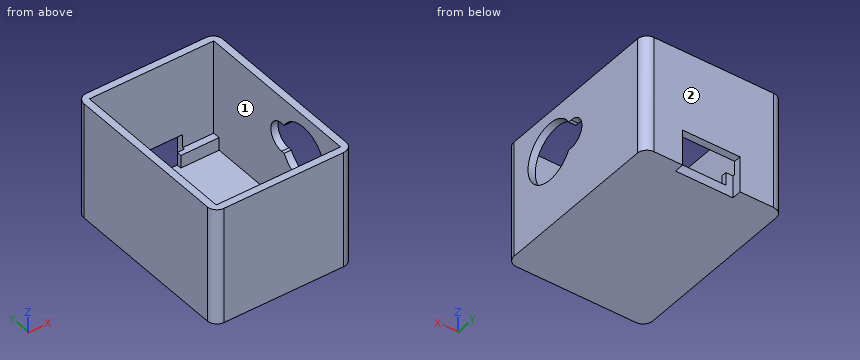
```python
from build123d import *

# Parameters (mm, degrees)
SKETCH_1_W               = 29
SKETCH_1_H               = 38.5
EXTRUDE_1_DEPTH          = 24
SHELL_1_T                = -1.5
SKETCH_7_W               = 26
SKETCH_7_H               = 5.5
EXTRUDE_7_DEPTH          = 2.5
SKETCH_5_W               = 2.7
SKETCH_5_H               = 1.5
EXTRUDE_8_DEPTH          = 8
SKETCH_6_W               = 2.7
SKETCH_6_H               = 1.5
EXTRUDE_9_DEPTH          = 9
SKETCH_9_W               = 29
SKETCH_9_H               = 38.5
EXTRUDE_10_DEPTH         = 0.5
FILLET_3_R               = 2
CUT_EXTRUDE_8_DEPTH      = 1.5
CUT_EXTRUDE_8_DEPTH_BACK = 7
SKETCH_2_W               = 12
SKETCH_2_H               = 2
SKETCH_10_R              = 3
SKETCH_10_R_2            = 6.072147162
CUT_EXTRUDE_9_DEPTH      = 1.5


with BuildPart() as part:
    # 草图1 → 凸台-拉伸1 (new body)
    with BuildSketch(Plane.XY):
        with Locations((14.5, -19.25)):
            Rectangle(SKETCH_1_W, SKETCH_1_H)
    extrude(amount=EXTRUDE_1_DEPTH)

    # 抽壳1
    shell_1_openings = [part.faces().sort_by_distance(p)[0] for p in [
        (14.5, -19.25, 24),
    ]]
    offset(amount=SHELL_1_T, openings=shell_1_openings, kind=Kind.INTERSECTION)

    # 草图7 → 凸台-拉伸7 (add)
    with BuildSketch(Plane.XY.offset(1.5)):
        with Locations((14.5, -34.25)):
            Rectangle(SKETCH_7_W, SKETCH_7_H)
    extrude(amount=EXTRUDE_7_DEPTH)

    # 草图5 → 凸台-拉伸8 (add)
    with BuildSketch(Plane.ZY.offset(-27.5)):
        with Locations((2.85, -2.25)):
            Rectangle(SKETCH_5_W, SKETCH_5_H)
    extrude(amount=EXTRUDE_8_DEPTH)

    # 草图6 → 凸台-拉伸9 (add)
    with BuildSketch(Plane(origin=(1.5, 0, 0), x_dir=(0, 0, -1), z_dir=(1, 0, 0))):
        with Locations((-2.85, -2.25)):
            Rectangle(SKETCH_6_W, SKETCH_6_H)
    extrude(amount=EXTRUDE_9_DEPTH)

    # 草图9 → 凸台-拉伸10 (add)
    with BuildSketch(Plane(origin=(0, 0, 0), x_dir=(-1, 0, 0), z_dir=(0, 0, -1))):
        with Locations((-14.5, -19.25)):
            Rectangle(SKETCH_9_W, SKETCH_9_H)
    extrude(amount=EXTRUDE_10_DEPTH)

    # 圆角3
    fillet_3_edges = [part.edges().sort_by_distance(p)[0] for p in [
        (0, 0, 11.75),
        (29, 0, 11.75),
        (29, -38.5, 11.75),
        (0, -38.5, 11.75),
    ]]
    fillet(fillet_3_edges, radius=FILLET_3_R)

    # 草图2 → 切除-拉伸8 (cut, two sides: drawn at the far end of the back side and taken through both)
    with BuildSketch(Plane(origin=(0, 0, 0), x_dir=(-1, 0, 0), z_dir=(0, 0, -1)).offset(-CUT_EXTRUDE_8_DEPTH_BACK)):
        with Locations((-15, -1)):
            Rectangle(SKETCH_2_W, SKETCH_2_H)
    extrude(amount=CUT_EXTRUDE_8_DEPTH + CUT_EXTRUDE_8_DEPTH_BACK, mode=Mode.SUBTRACT)

    # 草图10 → 切除-拉伸9 (cut)
    with BuildSketch(Plane(origin=(29, 0, 0), x_dir=(0, 0, -1), z_dir=(1, 0, 0))):
        with Locations((-15.5, -20.5)):
            Circle(SKETCH_10_R)
        with Locations((-15.5, -26.5)):
            Circle(SKETCH_10_R_2)
        with BuildLine():
            ThreePointArc((-18.422516621, -21.177419071), (-18.48056621, -20.840917978), (-18.5, -20.5))
            Line((-18.5, -20.5), (-18.5, -21.220703536))
            ThreePointArc((-18.5, -21.220703536), (-18.461337395, -21.198919734), (-18.422516621, -21.177419071))
        make_face()
        with BuildLine():
            Line((-12.5, -21.220703536), (-12.5, -20.5))
            ThreePointArc((-12.5, -20.5), (-12.51943379, -20.840917978), (-12.577483379, -21.177419071))
            ThreePointArc((-12.577483379, -21.177419071), (-12.538662605, -21.198919734), (-12.5, -21.220703536))
        make_face()
    extrude(amount=-CUT_EXTRUDE_9_DEPTH, mode=Mode.SUBTRACT)


solid = part.part
```
The listing builds one solid part. Answer for the finished solid, in the listing's coordinates (mm). Face numbers are marked on the shaded views. A direction names the side the tool comes from. Coordinates: 2 decimals unless noted, no trailing zeros. Write each loop counter-clockwise with the first axis right and the second up, starting at its lowest first coordinate (ties: lowest second). Pieces come first, ordered by that corner, then holes. Notation, with made-up numbers: (51, -14.5) - (77, -14.5) arc R27 ccw to (77, 14.5) - close; hole circle Ø7 at (44.5, 8.5). An arc over 180 degrees is marked (long way). Return JSON: item names as keys, results as strings. Group by question number.
Q1. Find the intervals of material crossed by line 1 along X through (y, z) = (-12, 3.5); line 2 along Y through (x, z) = (15, 11.5); line 3 along Z through (x, y) = (27.9, -26.5), in increasing order. Write a range as [from, to].
Q2. Flat-ended cylindrical pins translate along their axes: pin 1 Ø0.8 at (x, y) = (15.5, -0.5) entering from -Z; pin 2 Ø1.6 at (y, z) = (-0.5, 3) entering from -X; pin 3 Ø5 at (x, z) = (13.5, 1) entering from +Y. Find the tip coordinate at first contact, or state that the pin passes through.
Q3. The part is cut by section A-A on y = -26.5. Write down the section's boundary in (x, z), and give its area (3 significant figures).
Q4. Which of the six approach directions +Z, -Z, +X, -X, +Y, -Y give full straight-line access (tool end or side, diameter ignored) to the marked faces 1 and 2?
Q5. The part is cut by section B-B on x = 15.25. Write down the section's boundary in (y, z), and give its area (3 significant figures).
Q6. The part is cut by section D-D on z = 15.5. Write down the section's boundary in (x, y), and give its area (3 significant figures).
Q7. The part is cut by section C-C on y = -33.5. Write down the section's boundary in (x, z).
Evaluation:
{
 "1": {"line 1": "x = [0, 1.5], [27.5, 29]", "line 2": "y = [-38.5, -37], [-1.5, 0]", "line 3": "z = [-0.5, 9.43], [21.57, 24]"},
 "2": {"pin 1": "stops at z = 7", "pin 2": "stops at x = 0.13", "pin 3": "stops at y = -2"},
 "3": {"outline": "(0, -0.5) - (29, -0.5) - (29, 9.43) - (27.5, 9.43) - (27.5, 1.5) - (1.5, 1.5) - (1.5, 24) - (0, 24) - close; (27.5, 21.57) - (29, 21.57) - (29, 24) - (27.5, 24) - close", "area": "107 mm2"},
 "4": {"face 1": "+Z", "face 2": "+Z, -Z, +X, -X, +Y"},
 "5": {"outline": "(-38.5, -0.5) - (-2, -0.5) - (-2, 1.5) - (-31.5, 1.5) - (-31.5, 4) - (-37, 4) - (-37, 24) - (-38.5, 24) - close; (-1.5, 7) - (0, 7) - (0, 24) - (-1.5, 24) - close", "area": "146 mm2"},
 "6": {"outline": "(0, -36.5) arc R2 ccw to (2, -38.5) - (27, -38.5) arc R2 ccw to (29, -36.5) - (29, -32.57) - (27.5, -32.57) - (27.5, -37) - (1.5, -37) - (1.5, -1.5) - (27.5, -1.5) - (27.5, -17.5) - (29, -17.5) - (29, -2) arc R2 ccw to (27, 0) - (2, 0) arc R2 ccw to (0, -2) - close", "area": "167 mm2"},
 "7": {"outline": "(0, -0.5) - (29, -0.5) - (29, 24) - (27.5, 24) - (27.5, 4) - (1.5, 4) - (1.5, 24) - (0, 24) - close"}
}
